Autodesk Inventor part; units mm, degrees
ref_plane "Start Plane" through (0, 0, 0) normal (0, 0, 1) x (1, 0, 0)
ref_plane "End Plane" through (0, 0, 440) normal (0, 0, 1) x (1, 0, 0)
ref_plane "Work Plane4" through (0, -20, 440) normal (0, 0.3827, 0.9239) x (1, 0, 0)
ref_plane "Start Plane" through (0, 0, 0) normal (0, 0, 1) x (1, 0, 0)
ref_plane "End Plane" through (0, 0, 440) normal (0, 0, 1) x (1, 0, 0)
sketch "Sketch" plane through (0, 0, 0) normal (0, 0, 1) x (1, 0, 0)
  line L0 (-20, -16) -> (-20, 16)
  line L1 (-16, 20) -> (16, 20)
  line L2 (20, 16) -> (20, -16)
  line L3 (16, -20) -> (-16, -20)
  arc A0 (-20, -16) -> (-16, -20) centre (-16, -16) ccw
  arc A1 (20, 16) -> (16, 20) centre (16, 16) ccw
  arc A2 (-16, 20) -> (-20, 16) centre (-16, 16) ccw
  arc A3 (16, -20) -> (20, -16) centre (16, -16) ccw
  arc A4 (-16, 18) -> (-18, 16) centre (-16, 16) ccw
  line L4 (-16, 18) -> (16, 18)
  arc A5 (18, 16) -> (16, 18) centre (16, 16) ccw
  line L5 (18, 16) -> (18, -16)
  arc A6 (16, -18) -> (18, -16) centre (16, -16) ccw
  line L6 (16, -18) -> (-16, -18)
  arc A7 (-18, -16) -> (-16, -18) centre (-16, -16) ccw
  line L7 (-18, -16) -> (-18, 16)
  line L8 (0, 29.1598) -> (0, -29.1598) construction
  line L9 (-29.1598, 0) -> (29.1598, 0) construction
  dimension "d7" = 4
  dimension "d9" = 40
  dimension "d11" = 40
  dimension "d12" = 2
  dimension "d15" = 20
  dimension "d16" = 20
extrude "Body" add sketch "Sketch" along normal up to surface (440 mm away) from surface at 0
sketch "Sketch3" plane through (0, 0, 0) normal (0, 0, 1) x (1, 0, 0)
  line L0 (0, 0) -> (10, 0)
ref_plane "Work Plane3" through (0, 0, 0) normal (0, -1, 0) x (1, 0, 0)
ref_plane "Work Plane4" through (0, -20, 440) normal (0, 0.3827, 0.9239) x (1, 0, 0)
split "Split1" plane through (0, -20, 440) removes the side toward (0, 0.3827, 0.9239)
sketch "Sketch4" plane through (0, 0, 0) normal (0, -1, 0) x (1, 0, 0)
  line L0 (-2, 0) -> (12, 0)
  line L1 (-2, 440) -> (12, 440)
  dimension "d18" = 440
equation "\"d7\" = G_IR"
equation "\"d9\" = G_W"
equation "\"d11\" = G_H"
equation "\"d12\" = G_T"
equation "\"d15\" = 0.5 * d9"
equation "\"d16\" = 0.5 * d11"
equation "\"d3\" = G_L"
equation "\"G_W\" = 40"
equation "\"G_H\" = 40"
equation "\"G_T\" = 2"
equation "\"G_IR\" = 4"
equation "\"G_L\" = d18"
equation "\"G_OFFSET_START\" = 0"
equation "\"G_OFFSET_END\" = 0"
properties part number "ISO 10799-2 - 40x40x2 - 440" material "Stainless Steel"
Could you check a few things on this model? Use its own coordinates, in mm. A direction names the side the tool comes from. Round coordinates to 2 decimals unless told otherwise and drop trailing zeros. Order: outer loops, then holes, each group sorted by start corner. A loop starts at its lowest first (then second) coordinate and runs counter-clockwise, first axis right, second up. Notation, with made-up numbers: M 9,34.25 L 41,34.25 A14 ccw 41,52.25 Z; hole C 12,13.5 d7. An arc over 180 degrees is marked long. One line per item, written item: value.
(1) I'm going to push a flat-ended pin straight in: P1, Ø12, axis at x = -8, y = -15, coming from the +Z side. Where does the tip first touch, or does it pass through?
Ans:
P1: stops at z = 440
(2) Which directions (+Z, -Z, +X, -X, +Y, -Y) give clear straight access to the entire face, cutting with the end or side of a thin tool? Please do faces 5 (the flat face through (0, -20, 217)), 6 (the flat face through (18, 0, 216)).
Ans:
face 5: +Z, -Z, +X, -X, -Y
face 6: +Z, -Z
(3) Imagine slicing it at B-B (z = 146.5). Write out the boundary of the cut face in (x, y), and give its area (3 significant figures).
Ans:
outline: M -20,-16 A4 ccw -16,-20 L 16,-20 A4 ccw 20,-16 L 20,16 A4 ccw 16,20 L -16,20 A4 ccw -20,16 Z; hole M -18,-16 A2 ccw -16,-18 L 16,-18 A2 ccw 18,-16 L 18,16 A2 ccw 16,18 L -16,18 A2 ccw -18,16 Z
area: 294 mm^2
(4) Imagine slicing it at C-C (y = -2). Write out the boundary of the cut face in (x, z).
Ans:
outline: M -20,0 L -18,0 L -18,432.54 L -20,432.54 Z; M 18,0 L 20,0 L 20,432.54 L 18,432.54 Z
(5) If we mould it in two halves opening along X, with no side actions, what happens to faces 1 (the flat face through (-18, 0, 216)), 2 (the flat face through (19.166, -1.575, 432.368)), 3 (the flat face through (20, 0, 216)), 4 (the flat face through (0, -18, 217))? For each: released by +X, released by -X, zero draft, split by the parting line, or undercut.
Ans:
face 1: undercut
face 2: zero draft
face 3: released by +X
face 4: undercut
(6) Imagine slicing it at A-A (x = -5). Write out the boundary of the cut face in (y, z), and give its area (3 significant figures).
Ans:
outline: M -20,0 L -18,0 L -18,439.17 L -20,440 Z; M 18,0 L 20,0 L 20,423.43 L 18,424.26 Z
area: 1,730 mm^2
(7) I need wall thicknesses on line 1 along X through (y, z) = (10, 421.5); line 2 along X through (y, z) = (17.5, 169). Which ranges of each line are inside material? Lowest first, please. Write a range as from..to.
Ans:
line 1: x = -20..-18, 18..20
line 2: x = -19.71..-17.32, 17.32..19.71
